Read the model definition and answer for the solid it produces. Units are mm, in the model's axes. A direction names the side the tool comes from. Give positions to 0.01 mm unless a question says otherwise; leave off trailing zeros. Loops run counter-clockwise (first coordinate to the right, second up) from the corner with the lowest first, then second, coordinate; pieces in that order, holes last. Notation, with made-up numbers: M 16.5,-11.75 L 68.5,-11.75 A20 cw 68.5,12.25 Z; hole C 51,-12 d3. An arc over 180 degrees is marked long. Return JSON: item names as keys, results as strings. Group by question number.
```python
from build123d import *
from build123d.topology import SkipClean

# Parameters (mm, degrees)
SKETCH_1_R               = 3
EXTRUDE_1_DEPTH          = 1.5
SKETCH_2_R               = 7
EXTRUDE_2_DEPTH          = 2
SKETCH_3_R               = 7
EXTRUDE_3_DEPTH          = 3
SKETCH_4_W               = 1
SKETCH_4_H               = 3
CUT_EXTRUDE_1_DEPTH      = 12.842719282
PATTERN_CIRCULAR_1_COUNT = 9
SKETCH_8_R               = 4
CUT_EXTRUDE_3_DEPTH      = 3
SKETCH_5_R               = 7
EXTRUDE_4_DEPTH          = 1
SKETCH_6_R               = 6
EXTRUDE_5_DEPTH          = 2
SKETCH_7_R               = 3.5
CUT_EXTRUDE_2_DEPTH      = 2
SKETCH_9_R               = 2.5
CUT_EXTRUDE_4_DEPTH      = 1


with BuildPart() as part:
    # 草图1 → 凸台-拉伸1 (new body)
    with BuildSketch(Plane(origin=(0, 0, 0), x_dir=(1, 0, 0), z_dir=(0, 1, 0))):
        with Locations(Location((0, 0, 0), (0, 0, 270))):
            Circle(SKETCH_1_R)
        with BuildLine():
            Line((-1.299038106, 0.75), (1.299038106, 0.75))
            ThreePointArc((1.299038106, 0.75), (0, -1.5), (-1.299038106, 0.75))
        make_face(mode=Mode.SUBTRACT)
    extrude(amount=EXTRUDE_1_DEPTH)

    # 草图2 → 凸台-拉伸2 (add)
    with SkipClean():  # the faces are left unmerged after this step: merging them gives an invalid solid
        with BuildSketch(Plane(origin=(0, 1.5, 0), x_dir=(1, 0, 0), z_dir=(0, 1, 0))):
            with Locations(Location((0, 0, 0), (0, 0, 270))):
                Circle(SKETCH_2_R)
            with BuildLine():
                Line((1.299038106, 0.75), (-1.299038106, 0.75))
                ThreePointArc((-1.299038106, 0.75), (0, -1.5), (1.299038106, 0.75))
            make_face(mode=Mode.SUBTRACT)
        extrude(amount=EXTRUDE_2_DEPTH)

    # 草图3 → 凸台-拉伸3 (add)
    with SkipClean():  # the faces are left unmerged after this step: merging them gives an invalid solid
        with BuildSketch(Plane(origin=(0, 3.5, 0), x_dir=(1, 0, 0), z_dir=(0, 1, 0))):
            with Locations(Location((0, 0, 0), (0, 0, 270))):
                Circle(SKETCH_3_R)
        extrude(amount=EXTRUDE_3_DEPTH)

    # 草图4 → 切除-拉伸1 (cut, symmetric)
    with SkipClean():  # the faces are left unmerged after this step: merging them gives an invalid solid
        with BuildSketch(Plane.XY):
            with Locations((0, 5)):
                Rectangle(SKETCH_4_W, SKETCH_4_H)
        cut_extrude_1 = extrude(amount=CUT_EXTRUDE_1_DEPTH, both=True, mode=Mode.SUBTRACT)

    # 阵列(圆周)1: 切除-拉伸1 ×9 about axis
    with SkipClean():  # the faces are left unmerged after this step: merging them gives an invalid solid
        pattern_circular_1_axis = Axis((0, 0, 0), (0, 1, 0))
        for i in range(1, PATTERN_CIRCULAR_1_COUNT):
            add(cut_extrude_1.rotate(pattern_circular_1_axis, i * 360 / PATTERN_CIRCULAR_1_COUNT), mode=Mode.SUBTRACT)

    # 草图8 → 切除-拉伸3 (cut)
    with SkipClean():  # the faces are left unmerged after this step: merging them gives an invalid solid
        with BuildSketch(Plane(origin=(0, 6.5, 0), x_dir=(1, 0, 0), z_dir=(0, 1, 0))):
            Circle(SKETCH_8_R)
        extrude(amount=-CUT_EXTRUDE_3_DEPTH, mode=Mode.SUBTRACT)

    # 草图5 → 凸台-拉伸4 (add)
    with BuildSketch(Plane(origin=(0, 6.5, 0), x_dir=(1, 0, 0), z_dir=(0, 1, 0))):
        with Locations(Location((0, 0, 0), (0, 0, 270))):
            Circle(SKETCH_5_R)
    extrude(amount=EXTRUDE_4_DEPTH)

    # 草图6 → 凸台-拉伸5 (add)
    with BuildSketch(Plane(origin=(0, 7.5, 0), x_dir=(1, 0, 0), z_dir=(0, 1, 0))):
        with Locations(Location((0, 0, 0), (0, 0, 270))):
            Circle(SKETCH_6_R)
    extrude(amount=EXTRUDE_5_DEPTH)

    # 草图7 → 切除-拉伸2 (cut)
    with BuildSketch(Plane(origin=(0, 9.5, 0), x_dir=(1, 0, 0), z_dir=(0, 1, 0))):
        with Locations(Location((0, 0, 0), (0, 0, 270))):
            Circle(SKETCH_7_R)
    extrude(amount=-CUT_EXTRUDE_2_DEPTH, mode=Mode.SUBTRACT)

    # 草图9 → 切除-拉伸4 (cut)
    with BuildSketch(Plane(origin=(0, 7.5, 0), x_dir=(1, 0, 0), z_dir=(0, 1, 0))):
        with Locations(Location((0, 0, 0), (0, 0, 270))):
            Circle(SKETCH_9_R)
    extrude(amount=-CUT_EXTRUDE_4_DEPTH, mode=Mode.SUBTRACT)


solid = part.part
```
1. The mould has two halves that part along Z. Classify faces 5 (the flat face through (0.5, 5, 5)), 6 (the flat face through (-5.326, 4.979, 1.447)), 7 (the flat face through (-4.97, 4.98, 2.29)), 8 (the cylindrical face through (0.9, 0.74, 2.86)): +Z half, -Z half, draft (parallel to the pull), parting line (faces both ways), or undercut.
2. Find section D-D (x = -5.5). Write down the section's boundary in (y, z), and give its area (3 significant figures).
3. For faces 1 (the cylindrical face through (-2.681, 3.125, 6.466)), 2 (the flat face through (-0.5, 5, 5)), 3 (the flat face through (-5.28, 4.98, -1.44)), 4 (the flat face through (4.51, 4.98, -3.18)), determine the directions among +Z, -Z, +X, -X, +Y, -Y from which every point of the face is accessible in a straight line to the end or side of a thin tool.
4. Find section C-C (y = 8). Write down the section's boundary in (x, z).
Result:
{
 "1": {"face 5": "draft", "face 6": "undercut", "face 7": "undercut", "face 8": "parting line"},
 "2": {"outline": "M 1.5,-4.33 L 7.5,-4.33 L 7.5,-2.4 L 9.5,-2.4 L 9.5,2.4 L 7.5,2.4 L 7.5,4.33 L 1.5,4.33 Z; hole M 3.5,-3.75 L 6.5,-3.75 L 6.5,-2.6 L 3.5,-2.6 Z; hole M 3.5,-1.48 L 6.5,-1.48 L 6.5,-0.46 L 3.5,-0.46 Z; hole M 3.5,0.46 L 6.5,0.46 L 6.5,1.48 L 3.5,1.48 Z; hole M 3.5,2.6 L 6.5,2.6 L 6.5,3.75 L 3.5,3.75 Z", "area": "48.5 mm2"},
 "3": {"face 1": "+Y, -Y", "face 2": "+Z, -Z", "face 3": "-X", "face 4": "none"},
 "4": {"outline": "C 0,0 d12; hole C 0,0 d7"}
}
